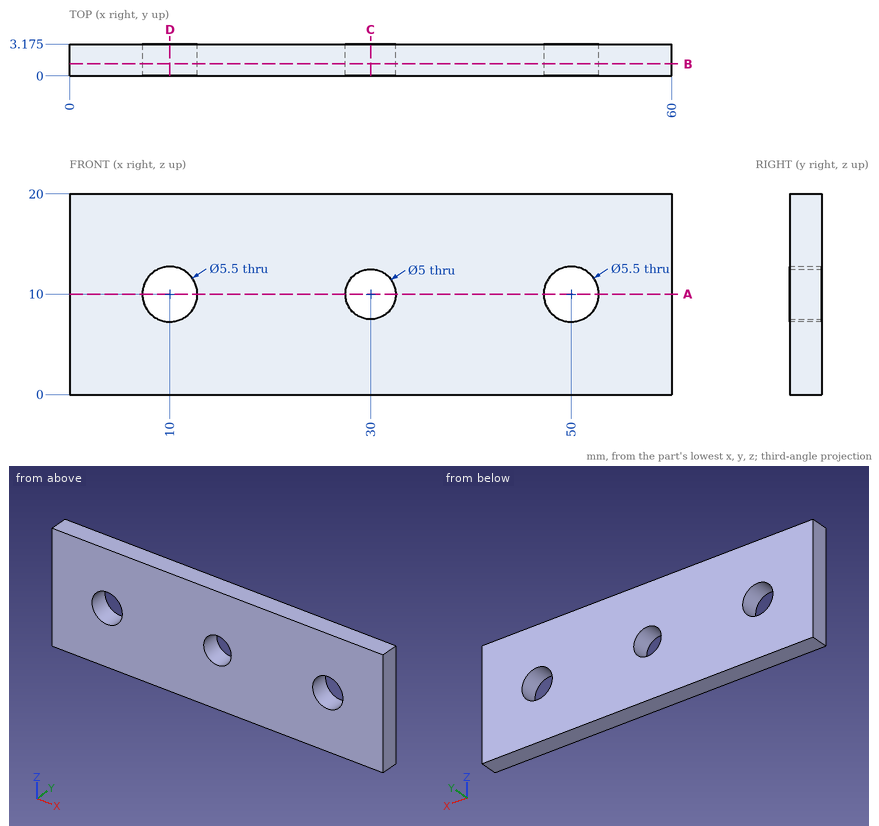
Print and shaded views of the part. All mm, measured from the part's lowest x, y and z. Give positions to 0.01 mm unless a question says otherwise; leave off trailing zeros. Order: outer loops, then holes, each group sorted by start corner. A loop starts at its lowest first (then second) coordinate and runs counter-clockwise, first axis right, second up. Notation, with made-up numbers: (30, 84.25) - (52, 84.25) arc R21 cw to (52, 110.25) - close; hole circle Ø9 at (54.5, -36). An arc over 180 degrees is marked (long way). One line per item, written item: value.
Item 1: Slice it at B-B (y = 1.2). List the corners of the cut face in (x, z), then the cut area to 3 significant figures.
Response values:
outline: (0, 0) - (60, 0) - (60, 20) - (0, 20) - close; hole circle Ø5.5 at (10, 10); hole circle Ø5 at (30, 10); hole circle Ø5.5 at (50, 10)
area: 1,130 mm2
Item 2: Slice it at D-D (x = 10). List the corners of the cut face in (y, z) (3 decimals).
Response values:
outline: (0, 0) - (3.175, 0) - (3.175, 7.25) - (0, 7.25) - close; (0, 12.75) - (3.175, 12.75) - (3.175, 20) - (0, 20) - close
Item 3: Wall check: line 1 (Z direction, x = 10, y = 1.75); line 2 (X direction, y = 0.95, z = 11.5); line 3 (X direction, y = 2.8, z = 9.5). Give the ranges that are in metal, low to high.
Response values:
line 1: 0 to 7.25, 12.75 to 20
line 2: 0 to 7.7, 12.3 to 28, 32 to 47.7, 52.3 to 60
line 3: 0 to 7.3, 12.7 to 27.55, 32.45 to 47.3, 52.7 to 60
Item 4: Slice it at A-A (z = 10). List the corners of the cut face in (x, y) (3 decimals).
Response values:
outline: (0, 0) - (7.25, 0) - (7.25, 3.175) - (0, 3.175) - close; (12.75, 0) - (27.5, 0) - (27.5, 3.175) - (12.75, 3.175) - close; (32.5, 0) - (47.25, 0) - (47.25, 3.175) - (32.5, 3.175) - close; (52.75, 0) - (60, 0) - (60, 3.175) - (52.75, 3.175) - close
Item 5: Slice it at C-C (x = 30). List the corners of the cut face in (y, z) (3 decimals).
Response values:
outline: (0, 0) - (3.175, 0) - (3.175, 7.5) - (0, 7.5) - close; (0, 12.5) - (3.175, 12.5) - (3.175, 20) - (0, 20) - close
